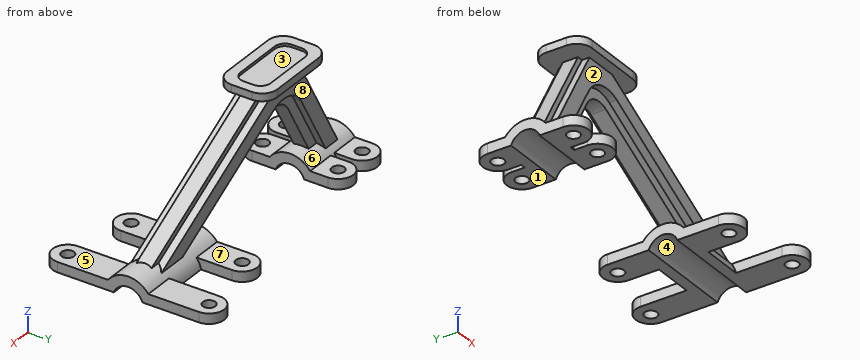
```python
from build123d import *

# Parameters (mm, degrees)
PAD_DEPTH         = 600
PAD001_DEPTH      = 15
PAD002_DEPTH      = 30
SKETCH004_W       = 270
SKETCH004_H       = 40
POCKET_DEPTH      = 48.990795
POCKET_DEPTH_BACK = -48.990795
PAD003_DEPTH      = 15
POCKET001_DEPTH   = 5
SKETCH007_R       = 12.5
PAD004_DEPTH      = 20


with BuildPart() as part:
    # Sketch (on YZ_Plane of Origin) → Pad (new body)
    with BuildSketch(Plane.YZ):
        with BuildLine():
            ThreePointArc((28.284271, 0), (0, 20), (-28.284271, 0))
            Line((-48.989795, 0), (-28.284271, 0))
            ThreePointArc((48.989795, 0), (0, 40), (-48.989795, 0))
            Line((28.284271, 0), (48.989795, 0))
        make_face()
    extrude(amount=PAD_DEPTH)

    # Sketch002 (on XZ_Plane of Origin) → Pad001 (join, symmetric)
    with BuildSketch(Plane.XZ):
        with BuildLine():
            Line((18.783308, 20), (130.950231, 220))
            Line((130.950231, 220), (229.049769, 220))
            Line((229.049769, 220), (585.661137, 20))
            Line((463.001241, 20), (585.661137, 20))
            Line((212.293102, 160.605803), (463.001241, 20))
            ThreePointArc((212.293102, 160.605803), (181.892852, 164.222858), (157.838985, 145.28428))
            Line((87.575223, 20), (157.838985, 145.28428))
            Line((18.783308, 20), (87.575223, 20))
        make_face()
    extrude(amount=PAD001_DEPTH, both=True)

    # Sketch003 → Pad002 (join, symmetric)
    with BuildSketch(Plane.XZ):
        with BuildLine():
            Line((30.248627, 20), (142.41555, 220))
            Line((142.41555, 220), (208.606453, 220))
            Line((208.606453, 220), (565.217821, 20))
            Line((565.217821, 20), (503.887873, 20))
            Line((503.887873, 20), (222.076251, 178.049713))
            ThreePointArc((222.076251, 178.049713), (176.475876, 183.475296), (140.395074, 155.067429))
            Line((140.395074, 155.067429), (64.644585, 20))
            Line((64.644585, 20), (30.248627, 20))
        make_face()
    pad002 = extrude(amount=PAD002_DEPTH, both=True)

    # Mirrored: Pad002 across XZ
    add(pad002.mirror(Plane.XZ))

    # Sketch004 (on XZ_Plane of Origin) → Pocket (cut, two sides)
    with BuildSketch(Plane.XZ) as pocket_sk:
        with Locations((265, 20)):
            Rectangle(SKETCH004_W, SKETCH004_H)
    extrude(amount=-POCKET_DEPTH, mode=Mode.SUBTRACT)
    extrude(pocket_sk.sketch, amount=-POCKET_DEPTH_BACK, mode=Mode.SUBTRACT)

    # Sketch005 (on Face27 of Pocket) → Pad003 (join)
    with BuildSketch(Plane.XY.offset(220)):
        with BuildLine():
            Line((90, 20), (90, -20))
            ThreePointArc((90, -20), (98.786797, -41.213203), (120, -50))
            Line((120, -50), (240, -50))
            ThreePointArc((240, -50), (261.213203, -41.213203), (270, -20))
            Line((270, -20), (270, 20))
            ThreePointArc((270, 20), (261.213203, 41.213203), (240, 50))
            Line((240, 50), (120, 50))
            ThreePointArc((120, 50), (98.786797, 41.213203), (90, 20))
        make_face()
    extrude(amount=PAD003_DEPTH)

    # Sketch006 (on Face45 of Pad003) → Pocket001 (cut)
    with BuildSketch(Plane.XY.offset(235)):
        with BuildLine():
            Line((110, 10), (110, -10))
            ThreePointArc((110, -10), (115.857864, -24.142136), (130, -30))
            Line((130, -30), (230, -30))
            ThreePointArc((230, -30), (244.142136, -24.142136), (250, -10))
            Line((250, -10), (250, 10))
            ThreePointArc((250, 10), (244.142136, 24.142136), (230, 30))
            Line((230, 30), (130, 30))
            ThreePointArc((130, 30), (115.857864, 24.142136), (110, 10))
        make_face()
    extrude(amount=-POCKET001_DEPTH, mode=Mode.SUBTRACT)

    # Sketch007 (on XY_Plane of Origin) → Pad004 (join)
    with BuildSketch(Plane.XY):
        with BuildLine():
            Line((0, -28.284271), (0, -75))
            ThreePointArc((0, -75), (30, -105), (60, -75))
            Line((60, -75), (60, -28.284271))
            Line((60, -28.284271), (0, -28.284271))
        make_face()
        with Locations((30, -75)):
            Circle(SKETCH007_R, mode=Mode.SUBTRACT)
        with BuildLine():
            Line((130, -28.284271), (130, -75))
            ThreePointArc((70, -75), (100, -105), (130, -75))
            Line((70, -75), (70, -28.284271))
            Line((70, -28.284271), (130, -28.284271))
        make_face()
        with Locations((100, -75)):
            Circle(SKETCH007_R, mode=Mode.SUBTRACT)
        with BuildLine():
            Line((400, -28.284271), (460, -28.284271))
            Line((460, -28.284271), (460, -110))
            ThreePointArc((400, -110), (430, -140), (460, -110))
            Line((400, -110), (400, -28.284271))
        make_face()
        with Locations((430, -110)):
            Circle(SKETCH007_R, mode=Mode.SUBTRACT)
        with BuildLine():
            Line((540, -28.284271), (540, -140))
            ThreePointArc((540, -140), (570, -170), (600, -140))
            Line((600, -140), (600, -28.284271))
            Line((600, -28.284271), (540, -28.284271))
        make_face()
        with Locations((570, -140)):
            Circle(SKETCH007_R, mode=Mode.SUBTRACT)
    pad004 = extrude(amount=PAD004_DEPTH)

    # Mirrored001: Pad004 across XZ
    add(pad004.mirror(Plane.XZ))


solid = part.part
```
Source: CAD feature listing. Evaluate the final solid. Frame: model axes, mm. Face numbers are marked on the shaded views. A direction names the side the tool comes from. Coordinates: 2 decimals unless noted, no trailing zeros. Write each loop counter-clockwise with the first axis right and the second up, starting at its lowest first coordinate (ties: lowest second). Pieces come first, ordered by that corner, then holes. Notation, with made-up numbers: (32.5, -24) -> (51.5, -24) arc R15 cw to (51.5, -12) -> close; hole circle Ø5 at (55.25, -30.5). An arc over 180 degrees is marked (long way). Return JSON: item names as keys, results as strings. Group by question number.
1) Section query D-D, the plane x = 151. Return loops of the section in (y, z).
2) Section query C-C, the plane z = 198. Return loops of the section in (x, y).
3) Set-up query: the marked faces 5, 6, 7 and 8. Return all of +Z, -Z, +X, -X, +Y, -Y with unobstructed straight access to the full face (end or side cutting, diameter ignored); none if empty.
4) Mould query, pull axis Y, two halves, no side actions, for the marked faces 1, 2, 3 and 4. Classes: +Y half, -Y half, draft (parallel to the pull), parting line (faces both ways), or undercut.
5) Section query B-B, the plane x = 308. Return loops of the section in (y, z).
6) Contact query for flat-ended pins moving along their axis: P1, Ø12, axis at x = 147.5, y = -33, coming from the -Z side; P2, Ø8, axis at y = 0.5, z = 77, coming from the +X side; P3, Ø4, axis at y = 4.5, z = 231.5, coming from the -X side. Output: stop coordinate, or through.
7) Ray query, line 1 along X through (y, z) = (75, 8.5); line 2 along Y through (x, z) = (30, 5); line 3 along Y through (x, z) = (30, 9). Return the intervals inside material, ascending.
8) Section query A-A, the plane z = 52. Return loops of the section in (x, y), plus the area to 3 significant figures.
From the geometry:
{
 "1": {"outline": "(-50, 220) -> (-30, 220) -> (-30, 168.83) -> (-15, 168.83) -> (-15, 133.09) -> (15, 133.09) -> (15, 168.83) -> (30, 168.83) -> (30, 220) -> (50, 220) -> (50, 235) -> (30, 235) -> (30, 230) -> (-30, 230) -> (-30, 235) -> (-50, 235) -> close"},
 "2": {"outline": "(118.61, -15) -> (130.08, -15) -> (130.08, -30) -> (247.83, -30) -> (247.83, -15) -> (268.28, -15) -> (268.28, 15) -> (247.83, 15) -> (247.83, 30) -> (130.08, 30) -> (130.08, 15) -> (118.61, 15) -> close"},
 "3": {"face 5": "+Z, +X, -X, -Y", "face 6": "none", "face 7": "+Z, +X, -X, +Y", "face 8": "+X, -X, +Y"},
 "4": {"face 1": "draft", "face 2": "-Y half", "face 3": "undercut", "face 4": "undercut"},
 "5": {"outline": "(-30, 129.86) -> (-15, 129.86) -> (-15, 106.93) -> (15, 106.93) -> (15, 129.86) -> (30, 129.86) -> (30, 164.26) -> (15, 164.26) -> (15, 175.72) -> (-15, 175.72) -> (-15, 164.26) -> (-30, 164.26) -> close"},
 "6": {"P1": "z = 158.24", "P2": "x = 491.16", "P3": "x = 90"},
 "7": {"line 1": "0 to 17.5, 42.5 to 60, 70 to 87.5, 112.5 to 130, 400 to 460, 540 to 600", "line 2": "-105 to -87.5, -62.5 to -25.98, 25.98 to 62.5, 87.5 to 105", "line 3": "-105 to -87.5, -62.5 to -23.22, 23.22 to 62.5, 87.5 to 105"},
 "8": {"outline": "(36.73, -15) -> (48.2, -15) -> (48.2, -30) -> (82.59, -30) -> (82.59, -15) -> (105.52, -15) -> (105.52, 15) -> (82.59, 15) -> (82.59, 30) -> (48.2, 30) -> (48.2, 15) -> (36.73, 15) -> close; (405.94, -15) -> (446.83, -15) -> (446.83, -30) -> (508.16, -30) -> (508.16, -15) -> (528.6, -15) -> (528.6, 15) -> (508.16, 15) -> (508.16, 30) -> (446.83, 30) -> (446.83, 15) -> (405.94, 15) -> close", "area": "8,620 mm²"}
}
